Study the drawing (mm; zero at the part's minimum x, y, z) and answer. Round coordinates to 2 decimals unless told otherwise and drop trailing zeros. Loops run counter-clockwise (first coordinate to the right, second up) from the corner with the lowest first, then second, coordinate; pieces in that order, holes last. Notation, with made-up numbers: (87.5, 78) -> (125.5, 78) arc R19 cw to (125.5, 98) -> close; hole circle Ø5 at (-9, -19.5). An arc over 180 degrees is marked (long way). Use one line per item in the form item = value.
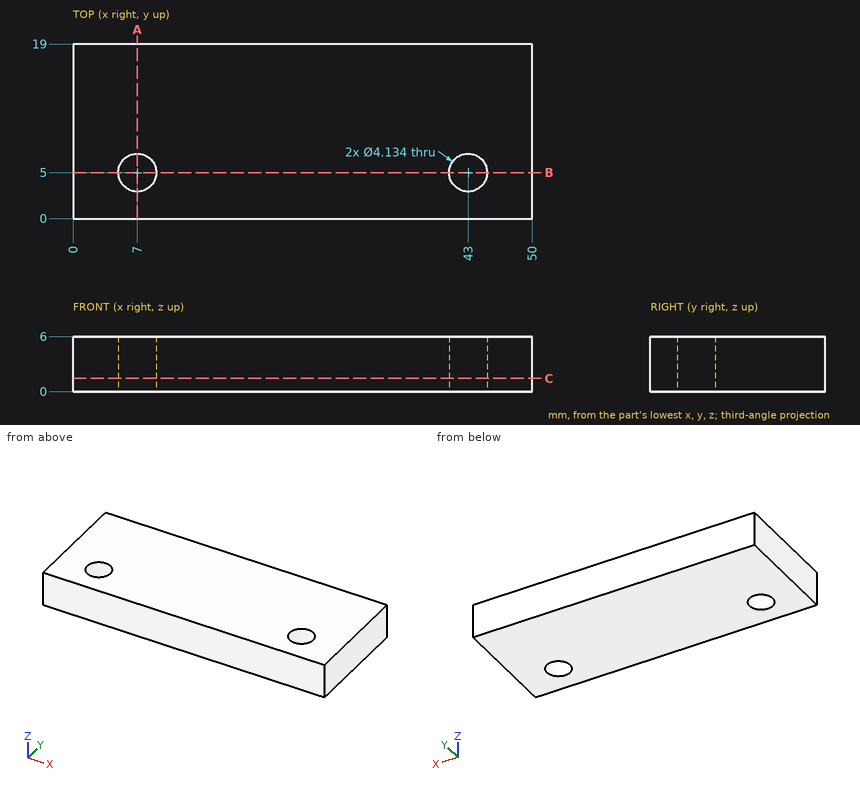
(1) Find section B-B, the plane y = 5. Write down the section's boundary in (x, z).
Completed:
outline = (0, 0) -> (4.93, 0) -> (4.93, 6) -> (0, 6) -> close; (9.07, 0) -> (40.93, 0) -> (40.93, 6) -> (9.07, 6) -> close; (45.07, 0) -> (50, 0) -> (50, 6) -> (45.07, 6) -> close
(2) Find section C-C, the plane z = 1.45. Write down the section's boundary in (x, y), then the cut area to 3 significant figures.
Completed:
outline = (0, 0) -> (50, 0) -> (50, 19) -> (0, 19) -> close; hole circle Ø4.13 at (7, 5); hole circle Ø4.13 at (43, 5)
area = 923 mm2
(3) Find section A-A, the plane x = 7. Write down the section's boundary in (y, z), then the cut area to 3 significant figures.
Completed:
outline = (0, 0) -> (2.93, 0) -> (2.93, 6) -> (0, 6) -> close; (7.07, 0) -> (19, 0) -> (19, 6) -> (7.07, 6) -> close
area = 89.2 mm2
(4) Consider L1, parallel to X at y = 5, z = 3.9; L2, parallel to Y at x = 43, z = 4.2; L3, parallel to Y at x = 44, z = 4.9. Determine where each line is inside the solid, lowest interval first.
Completed:
L1 = 0 to 4.93, 9.07 to 40.93, 45.07 to 50
L2 = 0 to 2.93, 7.07 to 19
L3 = 0 to 3.19, 6.81 to 19
